from build123d import *

# Parameters (mm, degrees)
SKETCH1_R                                    = 8
BOSS_EXTRUDE1_DEPTH                          = 3
CSK_FOR_M3_COUNTERSUNK_FLAT_HEAD_SCR_2_COUNT = 2
CSK_FOR_M3_COUNTERSUNK_FLAT_HEAD_SCR_2_PITCH = 30
CSK_FOR_M3_COUNTERSUNK_FLAT_HEAD_SCR_3_COUNT = 2
CSK_FOR_M3_COUNTERSUNK_FLAT_HEAD_SCR_3_PITCH = 42.426406871
CSK_FOR_M3_COUNTERSUNK_FLAT_HEAD_SCR_4_COUNT = 2
CSK_FOR_M3_COUNTERSUNK_FLAT_HEAD_SCR_4_PITCH = 30
CHAMFER1_SIZE                                = 2
BOSS_EXTRUDE2_DEPTH                          = 1.75


with BuildPart() as part:
    # Sketch1 → Boss-Extrude1 (new body)
    with BuildSketch(Plane(origin=(0, 0, 0), x_dir=(1, 0, 0), z_dir=(0, 1, 0))):
        with BuildLine():
            Line((-15, -15), (15, -15))
            ThreePointArc((15, -15), (18.535533906, -13.535533906), (20, -10))
            Line((20, -10), (20, 20))
            ThreePointArc((20, 20), (18.535533906, 23.535533906), (15, 25))
            Line((15, 25), (-15, 25))
            ThreePointArc((-15, 25), (-18.535533906, 23.535533906), (-20, 20))
            Line((-20, 20), (-20, -10))
            ThreePointArc((-20, -10), (-18.535533906, -13.535533906), (-15, -15))
        make_face()
        Circle(SKETCH1_R, mode=Mode.SUBTRACT)
    extrude(amount=-BOSS_EXTRUDE1_DEPTH)

    # Sketch6 → CSK for M3 Countersunk Flat Head Screw1 (revolve, cut)
    with BuildSketch(Plane(origin=(-15, 0, -20), x_dir=(0, 0, 1), z_dir=(1, 0, 0))):
        Polygon((0, 0), (0, 3), (1.7, 3), (1.7, 1.45), (3.15, 0), align=None)
    csk_for_m3_countersunk_flat_head_screw1 = revolve(axis=Axis((-15, 6.35, -20), (0, -1, 0)), mode=Mode.SUBTRACT)

    # CSK for M3 Countersunk Flat Head Scr 2: CSK for M3 Countersunk Flat Head Screw1 ×2
    with Locations(*[(i * CSK_FOR_M3_COUNTERSUNK_FLAT_HEAD_SCR_2_PITCH, 0, 0) for i in range(1, CSK_FOR_M3_COUNTERSUNK_FLAT_HEAD_SCR_2_COUNT)]):
        add(csk_for_m3_countersunk_flat_head_screw1, mode=Mode.SUBTRACT)

    # CSK for M3 Countersunk Flat Head Scr 3: CSK for M3 Countersunk Flat Head Screw1 ×2
    with Locations(*[Vector(0.707106781, 0, 0.707106781) * (i * CSK_FOR_M3_COUNTERSUNK_FLAT_HEAD_SCR_3_PITCH) for i in range(1, CSK_FOR_M3_COUNTERSUNK_FLAT_HEAD_SCR_3_COUNT)]):
        add(csk_for_m3_countersunk_flat_head_screw1, mode=Mode.SUBTRACT)

    # CSK for M3 Countersunk Flat Head Scr 4: CSK for M3 Countersunk Flat Head Screw1 ×2
    with Locations(*[(0, 0, i * CSK_FOR_M3_COUNTERSUNK_FLAT_HEAD_SCR_4_PITCH) for i in range(1, CSK_FOR_M3_COUNTERSUNK_FLAT_HEAD_SCR_4_COUNT)]):
        add(csk_for_m3_countersunk_flat_head_screw1, mode=Mode.SUBTRACT)

    # Chamfer1
    chamfer1_edges = [part.edges().sort_by_distance(p)[0] for p in [
        (-8, -3, 0),
    ]]
    chamfer(chamfer1_edges, length=CHAMFER1_SIZE)

    # Sketch9 → Boss-Extrude2 (add, symmetric)
    with BuildSketch(Plane(origin=(0, 0, 0), x_dir=(0, 0, -1), z_dir=(1, 0, 0))):
        Polygon((8, 0), (8, 15), (28, 15), (28, 9), (16, 9), (16, 0), align=None)
    extrude(amount=BOSS_EXTRUDE2_DEPTH, both=True)


solid = part.part
Part model, mm, in its own coordinate system. A direction names the side the tool comes from. Round coordinates to 2 decimals unless told otherwise and drop trailing zeros. Order: outer loops, then holes, each group sorted by start corner. A loop starts at its lowest first (then second) coordinate and runs counter-clockwise, first axis right, second up. Notation, with made-up numbers: (31.5, -21) -> (86.5, -21) arc R29 ccw to (86.5, 1) -> close; hole circle Ø9 at (-20.75, 38.5). An arc over 180 degrees is marked (long way). Put each result on its own line as item: value.
Q1. Band-saw the part on A-A (z = 0). Give the cut face in (x, y), and give its area (3 significant figures).
From the geometry:
outline: (-20, -3) -> (-10, -3) -> (-8, -1) -> (-8, 0) -> (-20, 0) -> close; (8, -1) -> (10, -3) -> (20, -3) -> (20, 0) -> (8, 0) -> close
area: 68.0 mm2
Q2. Band-saw the part on B-B (y = 5.75). Give the cut face in (x, z).
From the geometry:
outline: (-1.75, -16) -> (1.75, -16) -> (1.75, -8) -> (-1.75, -8) -> close
Q3. Pin check, flat tips, straight feed: pin 1 Ø20 at (x, z) = (9, 3.5) entering from +Y; pin 2 Ø1 at (x, y) = (0.5, 3) entering from -Z; pin 3 Ø4 at (x, y) = (-1, 8.5) entering from +Z. Stop position of each tip, or through.
From the geometry:
pin 1: stops at y = 0
pin 2: stops at z = -16
pin 3: stops at z = -8
Q4. Tool access for faces 5 (the face through (1.75, 9.3, -15.9)), 6 (the face through (-14.35, -2.21, -18.43)): list every direction of +Z, -Z, +X, -X, +Y, -Y with a clear straight run to the whole face (end or side of a thin tool).
From the geometry:
face 5: +Z, -Z, +X, +Y
face 6: +Y, -Y
Q5. Band-saw the part on D-D (y = 10.75). Give the cut face in (x, z).
From the geometry:
outline: (-1.75, -28) -> (1.75, -28) -> (1.75, -8) -> (-1.75, -8) -> close
Q6. Band-saw the part on C-C (z = -19). State how many separate pieces and enclosed holes the cut face has, and give its area (3 significant figures).
From the geometry:
separate pieces: 4
enclosed holes: 0
area: 120 mm2
Q7. Wall check: line 1 (Z direction, x = 15, y = -2.3); line 2 (X direction, y = -2, z = -20); line 3 (Z direction, x = 0, y = -0.65). Give the ranges that are in metal, low to high. Write a range as [from, to].
From the geometry:
line 1: z = [-25, -21.7], [-18.3, 8.3], [11.7, 15]
line 2: x = [-20, -16.7], [-13.3, 13.3], [16.7, 20]
line 3: z = [-25, -8], [8, 15]
Q8. Pull direction Z, two halves, no side cores. Call faces 1 (the face through (0, 5, -16)), 2 (the face through (0, -1, 15)), 3 (the face through (-13.5, -2.2, 10.8)), 4 (the face through (0, 9, -22)): pulls with the +Z half, pulls with the -Z half, needs draft (parallel to the pull), parting line crosses it, or undercut.
From the geometry:
face 1: pulls with the -Z half
face 2: pulls with the +Z half
face 3: undercut
face 4: needs draft
